Autodesk Inventor part; units mm, degrees
ref_plane "YZ Plane" through (0, 0, 0) normal (1, 0, 0) x (0, 1, 0)
ref_plane "XZ Plane" through (0, 0, 0) normal (0, 1, 0) x (-1, 0, 0)
ref_plane "XY Plane" through (0, 0, 0) normal (0, 0, 1) x (1, 0, 0)
sketch "Sketch5" plane through (0, 0, 0) normal (0, 0, 1) x (1, 0, 0)
  line L0 (52.8, -15.6) -> (52.8, -10.6)
  line L1 (52.8, -10.6) -> (49.8, -10.6)
  line L2 (49.8, -10.6) -> (49.8, -12.55)
  line L3 (44, -12.55) -> (44, -3.05)
  line L4 (49.8, -3.05) -> (49.8, -5)
  line L5 (49.8, -5) -> (52.8, -5)
  line L6 (52.8, -5) -> (52.8, 0)
  line L7 (52.8, 0) -> (7.8, 0)
  line L8 (44, -3.05) -> (49.8, -3.05)
  line L9 (44, -12.55) -> (49.8, -12.55)
  line L10 (52.8, -15.6) -> (7.8, -15.6)
  arc A0 (7.8, 0) -> (7.8, -15.6) centre (7.8, -7.8) ccw
  point P0 (0, 0)
  dimension "d41" = 5.8
  dimension "d48" = 44
  dimension "d50" = 3
  dimension "d63" = 45
  dimension "d67" = 15.6
  dimension "d71" = 0
  dimension "d72" = 36.2
  dimension "d87" = 5.6
  dimension "d88" = 9.5
extrude "Extrusion2" add sketch "Sketch5" along normal blind 12
sketch "Sketch11" plane through (0, 0, 12) normal (0, 0, 1) x (1, 0, 0)
  line L0 (52.8, 0) -> (7.8, 0)
  line L1 (9.0635, 0) -> (9.9318, -4.924)
  line L2 (9.9318, -4.924) -> (0.0837, -6.6605)
  arc A0 (7.8, 0) -> (7.8, -15.6) centre (7.8, -7.8) ccw
  point P0 (0, 0)
  dimension "d95" = 100
  dimension "d96" = 5
  dimension "d97" = 10
extrude "Extrusion7" cut sketch "Sketch11" along normal blind 8 from surface at -12
sketch "Sketch14" plane through (0, 0, 12) normal (0, 0, 1) x (1, 0, 0)
  line L0 (2.6339, 4.7908) -> (6.9247, -19.5432)
  line L1 (6.9247, -19.5432) -> (-9.4392, -22.4286)
  line L2 (-9.4392, -22.4286) -> (-13.7299, 1.9055)
  line L3 (-13.7299, 1.9055) -> (2.6339, 4.7908)
  line L4 (9.0635, 0) -> (9.9318, -4.924)
  point P0 (0, 0)
  dimension "d107" = 5.5
extrude "Extrusion10" cut sketch "Sketch14" against normal through all
fillet "Fillet2" radius 15 1 edges at (6.2001, -15.4342, 6)
equation "\"l1\" = 8"
properties part number "Finray_test_8_Kerbe_10deg_V4_links"
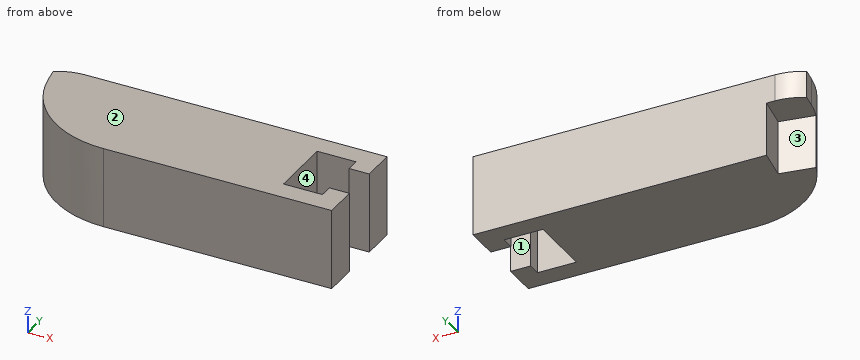
Geometry check sheet. Reference: the model listing, model coordinates, mm. Face numbers are marked on the shaded views. A direction names the side the tool comes from. Give positions to 0.01 mm unless a question says otherwise; leave off trailing zeros. Order: outer loops, then holes, each group sorted by start corner. A loop starts at its lowest first (then second) coordinate and runs counter-clockwise, first axis right, second up. Notation, with made-up numbers: (80, 0) - (100, 0) arc R14 cw to (100, 17) - close; hole circle Ø2 at (20.25, -6). An arc over 180 degrees is marked (long way). Answer as a JSON object with one key per item and string values.
(1) Tool access check on the marked faces 1, 2, 3 and 4. Record the directions out of +Z, -Z, +X, -X, +Y, -Y that give a thin tool (end or side, any length) a straight path to the whole face; none if there is none.
Report:
{"face 1": "+Z, -Z, +X", "face 2": "+Z, +X, -X, +Y, -Y", "face 3": "-Z, -X", "face 4": "+Z, -Z"}
(2) Cross-section at A-A (y = -3.75). Record the cut outline in (x, z).
Report:
{"outline": "(4.15, 8) - (9.72, 8) - (9.72, 0) - (44, 0) - (44, 12) - (4.15, 12) - close; (49.8, 0) - (52.8, 0) - (52.8, 12) - (49.8, 12) - close"}
(3) Material ranges on line 1 (Y direction, x = 48, z = 10); line 2 (X direction, y = -11.5, z = 8); line 3 (Y direction, x = 16, z = 4), recorded low to high.
Report:
{"line 1": "-15.6 to -12.55, -3.05 to 0", "line 2": "8.51 to 44, 49.8 to 52.8", "line 3": "-15.33 to 0"}
(4) Cross-section at D-D (y = -12). Record the cut outline in (x, z).
Report:
{"outline": "(9.07, 0) - (44, 0) - (44, 12) - (9.07, 12) - close; (49.8, 0) - (52.8, 0) - (52.8, 12) - (49.8, 12) - close"}
(5) Cross-section at B-B (z = 6.25). Record the cut outline in (x, y).
Report:
{"outline": "(4.76, -5.84) arc R15 ccw to (18.82, -15.6) - (52.8, -15.6) - (52.8, -10.6) - (49.8, -10.6) - (49.8, -12.55) - (44, -12.55) - (44, -3.05) - (49.8, -3.05) - (49.8, -5) - (52.8, -5) - (52.8, 0) - (9.06, 0) - (9.93, -4.92) - close"}
(6) Cross-section at C-C (x = 9.5). Record the cut outline in (y, z).
Report:
{"outline": "(-12.36, 0) - (-5, 0) - (-5, 8) - (-2.48, 8) - (-2.48, 0) - (0, 0) - (0, 12) - (-12.36, 12) - close"}
(7) Depth check by flat-ended pin: pin 1 Ø0.6 at (y, z) = (-4, 8.5) entering from -X; pin 2 Ø3 at (y, z) = (-8.5, 6.5) entering from +X; pin 3 Ø1.6 at (y, z) = (-12, 8) entering from -X. Enter the tip coordinate at first touch or a pass-through.
Report:
{"pin 1": "x = 4.14", "pin 2": "x = 44", "pin 3": "x = 8.2"}
